Check sheet for the modelled part. Datum: model origin and axes. Units: mm. Give positions to 0.01 mm unless a question says otherwise; leave off trailing zeros. Write each loop counter-clockwise with the first axis right and the second up, starting at its lowest first coordinate (ties: lowest second). Pieces come first, ordered by that corner, then holes. Notation, with made-up numbers: (22, 76.25) - (41, 76.25) arc R31 cw to (41, 104.25) - close; hole circle Ø7 at (36.5, -31.5). An arc over 180 degrees is marked (long way). Return JSON: item names as keys, results as strings. Group by question number.
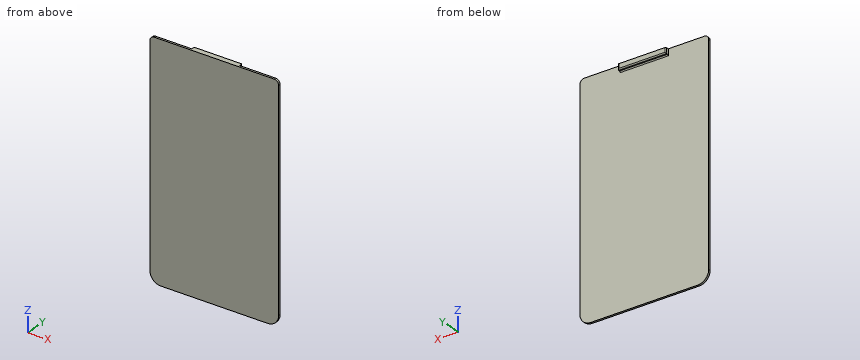
```python
from build123d import *

# Parameters (mm, degrees)
SKETCH2_W           = 59
SKETCH2_H           = 105
BOSS_EXTRUDE1_DEPTH = 0.925
SKETCH3_W           = 22
SKETCH3_H           = 2.5
BOSS_EXTRUDE2_DEPTH = 1.5
FILLET1_R           = 0.5
FILLET2_R           = 2
FILLET3_R           = 5


with BuildPart() as part:
    # Sketch2 → Boss-Extrude1 (new body)
    with BuildSketch(Plane(origin=(0, 0, 0), x_dir=(1, 0, 0), z_dir=(0, 1, 0))):
        with Locations((-29.5, 52.5)):
            Rectangle(SKETCH2_W, SKETCH2_H)
    extrude(amount=BOSS_EXTRUDE1_DEPTH)

    # Sketch3 → Boss-Extrude2 (add)
    with BuildSketch(Plane(origin=(0, 0.925, 0), x_dir=(1, 0, 0), z_dir=(0, 1, 0))):
        with Locations((-29.5, 1.25)):
            Rectangle(SKETCH3_W, SKETCH3_H)
    extrude(amount=BOSS_EXTRUDE2_DEPTH)

    # Fillet1
    fillet1_edges = [part.edges().sort_by_distance(p)[0] for p in [
        (-29.5, 0.925, -2.5),
        (-40.5, 2.425, -1.25),
        (-18.5, 2.425, -1.25),
        (-29.5, 2.425, -2.5),
    ]]
    fillet(fillet1_edges, radius=FILLET1_R)

    # Fillet2
    fillet2_edges = [part.edges().sort_by_distance(p)[0] for p in [
        (0, 0.4625, 0),
        (-59, 0.4625, 0),
    ]]
    fillet(fillet2_edges, radius=FILLET2_R)

    # Fillet3
    fillet3_edges = [part.edges().sort_by_distance(p)[0] for p in [
        (-59, 0.4625, -105),
        (0, 0.4625, -105),
    ]]
    fillet(fillet3_edges, radius=FILLET3_R)


solid = part.part
```
Item 1: Section check B-B on z = -81. Record the cut outline in (x, y) (3 decimals).
Item 2: Depth check by flat-ended pin: pin 1 (1 mm diameter, centred on x = -34, z = -38.5, fed in from +Y) (3 decimals). Enter the tip coordinate at first touch or a pass-through.
Item 3: Material ranges on line 1 along Y through (x, z) = (-10.5, -60) (3 decimals); line 2 along Z through (x, y) = (-37.5, 1.4); line 3 along Z through (x, y) = (-3.5, 0.7), recorded low to high. Write a range as from..to.
Item 4: Section check C-C on x = -52. Record the cut outline in (y, z) (3 decimals).
Item 5: Section check A-A on x = -20.5. Record the cut outline in (y, z) (3 decimals).
Reply:
{
 "1": {"outline": "(-59, 0) - (0, 0) - (0, 0.925) - (-59, 0.925) - close"},
 "2": {"pin 1": "y = 0.925"},
 "3": {"line 1": "0..0.925", "line 2": "-2.5..0", "line 3": "-104.77..0"},
 "4": {"outline": "(0, -105) - (0.925, -105) - (0.925, 0) - (0, 0) - close"},
 "5": {"outline": "(0, -105) - (0.925, -105) - (0.925, -3) arc R0.5 cw to (1.425, -2.5) - (1.925, -2.5) arc R0.5 ccw to (2.425, -2) - (2.425, 0) - (0, 0) - close"}
}
